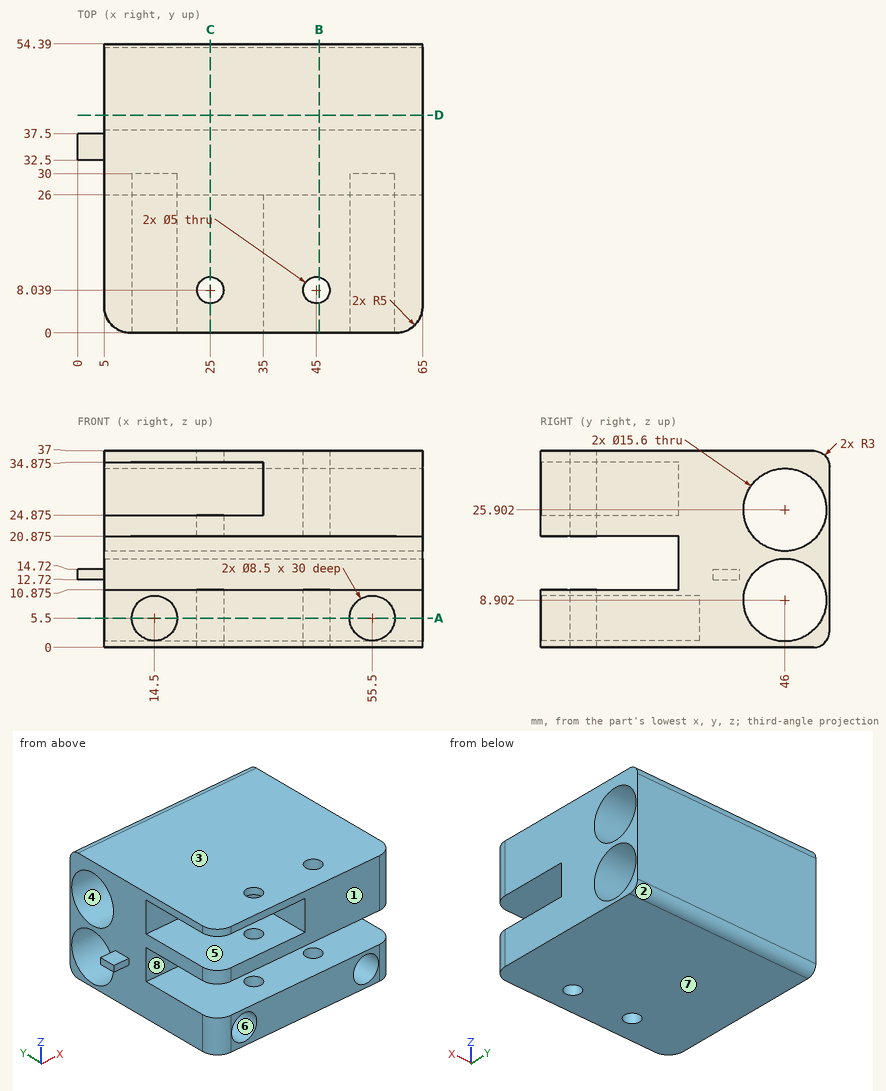
The figure shows three views and two pictorial views of one solid part (mm, origin at its lowest corner). Answer the questions. A direction names the side the tool comes from. Give positions to 0.01 mm unless a question says otherwise; leave off trailing zeros. Loops run counter-clockwise (first coordinate to the right, second up) from the corner with the lowest first, then second, coordinate; pieces in that order, holes last. Notation, with made-up numbers: (52.25, 78) -> (77.25, 78) arc R22 ccw to (77.25, 97) -> close; hole circle Ø4 at (4.5, 6). An arc over 180 degrees is marked (long way). Put each result on its own line as item: value. Start each with the question number.
Item 1: The part is cut by section A-A (z = 5.5). Give the vertices of the cut face in (x, y), then the cut area to 3 significant figures.
Item 2: The part is cut by section B-B (x = 45.5). Give the vertices of the cut face in (y, z) (1 decimal), then the cut area to 3 significant figures.
Item 3: Each of these flat-tipped pins is pushed along its axis until it touches: P1, Ø13, axis at x = 39, y = 10.5, coming from the -Z side; P2, Ø1.6, axis at x = 3.5, z = 14, coming from the -Y side; P3, Ø3, axis at x = 45, y = 8.04, coming from the -Z side; P4, Ø8, axis at x = 23.5, z = 15.5, coming from the -Y side. Where does it stop, or does it pass through?
Item 4: The part is cut by section C-C (x = 25). Give the vertices of the cut face in (y, z) (1 decimal).
Item 5: Find the intervals of material crossed by L1, parallel to Z at x = 33.5, y = 5.5 (1 decimal); L2, parallel to Z at x = 17, y = 25.5 (1 decimal); L3, parallel to Z at x = 9, y = 39.5 (1 decimal), in increasing order. Write a range as [from, to].
Item 6: The part is cut by section D-D (y = 41). Give the vertices of the cut face in (x, z) (1 decimal).
Item 7: The mould has two halves that part along Y. Classify the marked faces 1, 2, 3 and 4: released by +Y, released by -Y, zero draft, split by the parting line, or undercut.
Item 8: Which of the six approach directions +Z, -Z, +X, -X, +Y, -Y give full straight-line access (tool end or side, diameter ignored) to the marked faces 5, 6, 7 and 8?
Answers below:
1. outline: (5, 5) arc R5 ccw to (10, 0) -> (10.25, 0) -> (10.25, 30) -> (18.75, 30) -> (18.75, 0) -> (51.25, 0) -> (51.25, 30) -> (59.75, 30) -> (59.75, 0) -> (60, 0) arc R5 ccw to (65, 5) -> (65, 38.98) -> (5, 38.98) -> close; (5, 53.02) -> (65, 53.02) -> (65, 54.39) -> (5, 54.39) -> close; hole circle Ø5 at (25, 8.04); hole circle Ø5 at (45, 8.04)
1. area: 1,860 mm2
2. outline: (0, 0) -> (5.6, 0) -> (5.6, 10.9) -> (0, 10.9) -> close; (0, 20.9) -> (5.6, 20.9) -> (5.6, 37) -> (0, 37) -> close; (10.5, 0) -> (51.4, 0) arc R3 ccw to (54.4, 3) -> (54.4, 34) arc R3 ccw to (51.4, 37) -> (10.5, 37) -> (10.5, 20.9) -> (26, 20.9) -> (26, 10.9) -> (10.5, 10.9) -> close; hole circle Ø15.6 at (46, 8.9); hole circle Ø15.6 at (46, 25.9)
2. area: 1,230 mm2
3. P1: z = 0
3. P2: y = 32.5
3. P3: through
3. P4: y = 26
4. outline: (0, 0) -> (5.5, 0) -> (5.5, 10.9) -> (0, 10.9) -> close; (0, 20.9) -> (5.5, 20.9) -> (5.5, 24.9) -> (0, 24.9) -> close; (0, 34.9) -> (5.5, 34.9) -> (5.5, 37) -> (0, 37) -> close; (10.5, 0) -> (51.4, 0) arc R3 ccw to (54.4, 3) -> (54.4, 34) arc R3 ccw to (51.4, 37) -> (10.5, 37) -> (10.5, 34.9) -> (26, 34.9) -> (26, 24.9) -> (10.5, 24.9) -> (10.5, 20.9) -> (26, 20.9) -> (26, 10.9) -> (10.5, 10.9) -> close; hole circle Ø15.6 at (46, 8.9); hole circle Ø15.6 at (46, 25.9)
5. L1: [0, 10.9], [20.9, 24.9], [34.9, 37]
5. L2: [0, 2.1], [8.9, 10.9], [20.9, 24.9], [34.9, 37]
5. L3: [0, 4.6], [13.2, 21.6], [30.2, 37]
6. outline: (5, 0) -> (65, 0) -> (65, 2.9) -> (5, 2.9) -> close; (5, 14.9) -> (65, 14.9) -> (65, 19.9) -> (5, 19.9) -> close; (5, 31.9) -> (65, 31.9) -> (65, 37) -> (5, 37) -> close
7. face 1: released by -Y
7. face 2: released by +Y
7. face 3: zero draft
7. face 4: undercut
8. face 5: -X, -Y
8. face 6: -Y
8. face 7: -Z, +X, -X, +Y, -Y
8. face 8: +X, -X, -Y
